Geometry check sheet. Reference: drawing and pictorial views, mm from the part's lowest x, y, z. A direction names the side the tool comes from. Give positions to 0.01 mm unless a question says otherwise; leave off trailing zeros. Loops run counter-clockwise (first coordinate to the right, second up) from the corner with the lowest first, then second, coordinate; pieces in that order, holes last. Notation, with made-up numbers: M 21.25,2 L 30.25,2 A28 ccw 30.25,33 Z; hole C 54,32 d6. An arc over 180 degrees is marked long. One line per question, with ' | ' between items. Start each with the question number.
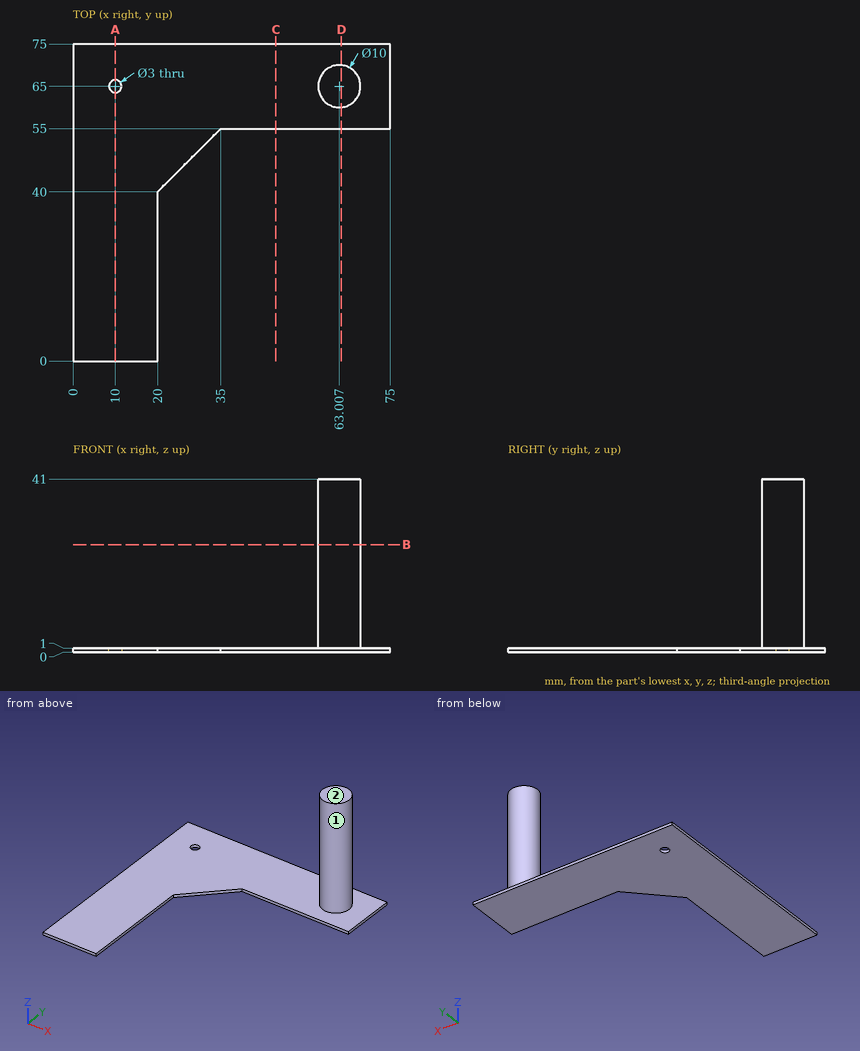
Q1. Material ranges on probe 1 along Y at (x, z) = (10, 0.3); probe 2 along Z at (x, y) = (37.5, 72); probe 3 along Y at (x, z) = (59.5, 4.5), recorded low to high. Write a range as from..to.
Q2. Cross-section at D-D (x = 63.5). Record the cut outline in (y, z), and give its area (3 significant figures).
Q3. Depth check by flat-ended pin: P1, Ø1.1, axis at x = 49.5, z = 0.5, coming from the -Y side; P2, Ø12, axis at x = 22.5, y = 19.5, coming from the +Z side; P3, Ø3, axis at x = 66, z = 5, coming from the +Y side. Enter the tip coordinate at first touch or a pass-through.
Q4. Cross-section at C-C (x = 48). Record the cut outline in (y, z).
Q5. Cross-section at A-A (x = 10). Record the cut outline in (y, z), and give its area (3 significant figures).
Q6. Cross-section at B-B (z = 25.5). Record the cut outline in (x, y), and give its area (3 significant figures).
Q7. Access from +Z, -Z, +X, -X, +Y, -Y to the whole of each face (thin tool, end or side, straight path). Record for the marked faces 1 and 2.
Solved:
1) probe 1: y = 0..63.5, 66.5..75 | probe 2: z = 0..1 | probe 3: y = 61.44..68.56
2) outline: M 55,0 L 75,0 L 75,1 L 69.98,1 L 69.98,41 L 60.02,41 L 60.02,1 L 55,1 Z | area: 418 mm²
3) P1: stops at y = 55 | P2: stops at z = 1 | P3: stops at y = 69.77
4) outline: M 55,0 L 75,0 L 75,1 L 55,1 Z
5) outline: M 0,0 L 63.5,0 L 63.5,1 L 0,1 Z; M 66.5,0 L 75,0 L 75,1 L 66.5,1 Z | area: 72.0 mm²
6) outline: C 63.01,65 d10 | area: 78.5 mm²
7) face 1: +Z | face 2: +Z, +X, -X, +Y, -Y
